```python
from build123d import *

# Parameters (mm, degrees)
F2_DEPTH = 12.7
F1_R     = 22.5055590266
F3_DEPTH = 7.62
F4_W     = 30.1420278847
F4_H     = 17.9640296847
F5_DEPTH = 2.54
F7_DEPTH = 1.27


with BuildPart() as f2:
    # F0 (on Front) → F2 (new body)
    with BuildSketch(Plane.XZ):
        Polygon((16.1803662777, 0), (37.0746999979, 0), (37.0746999979, 26.1179152876), (34.0169928968, 32.2333276272), (31.2140900642, 39.1131713986), (31.2140900642, 43.4449203312), (21.7861626297, 43.4449203312), (21.7861626297, 39.1131713986), (18.7284555286, 32.2333276272), (16.1803662777, 26.1179152876), align=None)
    extrude(amount=F2_DEPTH)


with BuildPart() as f3:
    # F1 (on Front) → F3 (new body)
    with BuildSketch(Plane.XZ):
        with Locations((78.2617554069, 32.2333276272)):
            Circle(F1_R)
    extrude(amount=F3_DEPTH)


with BuildPart() as f5:
    # F4 (on Top) → F5 (new body)
    with BuildSketch(Plane.XY):
        with Locations((-15.0710139424, 8.9820148423)):
            Rectangle(F4_W, F4_H)
    extrude(amount=F5_DEPTH)

    # F6 (on face) → F7 (join)
    with BuildSketch(Plane.XY.offset(2.54)):
        Polygon((-35.7478260994, 4.4591561891), (-30.1420278847, 2.4206847884), (0, 2.4206847884), (2.9831291176, 2.4206847884), (5.0216042437, 4.4591561891), (5.0216042437, 7.2620538995), (2.9831291176, 7.2620538995), (0, 7.2620538995), (-30.1420278847, 7.2620538995), (-32.6901189983, 7.2620538995), (-35.7478260994, 7.2620538995), align=None)
        Polygon((-30.1420278847, 11.8486145511), (0, 11.8486145511), (2.9831291176, 11.8486145511), (5.0216042437, 14.396703802), (0, 14.396703802), (-30.1420278847, 14.396703802), (-32.6901189983, 14.396703802), (-32.6901189983, 11.8486145511), align=None)
    extrude(amount=F7_DEPTH)


with BuildPart() as f12:
    # F11 (on Front) → F12 (revolve)
    with BuildSketch(Plane.XZ):
        with BuildLine():
            Line((0, -66.4687156677), (0, 55.9921823442))
            Line((0, 55.9921823442), (-22.0337584615, 55.9921823442))
            Line((-22.0337584615, 55.9921823442), (-35.9484543807, 45.556163555))
            ThreePointArc((-35.9484543807, 45.556163555), (-37.8180675739, 43.3159697459), (-38.4884551167, 40.476163003))
            Line((-38.4884551167, 40.476163003), (-38.4884551167, 26.2577953691))
            ThreePointArc((-38.4884551167, 26.2577953691), (-37.8180675121, 23.4179885028), (-35.9484541599, 21.1777946515))
            Line((-35.9484541599, 21.1777946515), (-32.1597233415, 18.3362476528))
            Line((-32.1597233415, 18.3362476528), (-37.2184558344, 11.5912683486))
            ThreePointArc((-37.2184558344, 11.5912683486), (-38.1625942485, 9.7893150524), (-38.4884551167, 7.7812693055))
            Line((-38.4884551167, 7.7812693055), (-38.4884551167, -21.9619643911))
            ThreePointArc((-38.4884551167, -21.9619643911), (-37.9697873011, -24.47554052), (-36.4985133985, -26.5784989984))
            Line((-36.4985133985, -26.5784989984), (-32.7925980091, -30.0785284489))
            Line((-32.7925980091, -30.0785284489), (-36.754989724, -34.2740041277))
            ThreePointArc((-36.754989724, -34.2740041277), (-38.0391963734, -36.2880546043), (-38.4884551167, -38.6340624095))
            Line((-38.4884551167, -38.6340624095), (-38.4884551167, -60.1187156677))
            ThreePointArc((-38.4884551167, -60.1187156677), (-36.6285831773, -64.6088437283), (-32.1384551167, -66.4687156677))
            Line((-32.1384551167, -66.4687156677), (0, -66.4687156677))
        make_face()
        with BuildLine():
            Line((0, 55.9921823442), (0, 67.4110209227))
            Line((0, 67.4110209227), (-20.4462584615, 67.4110209227))
            ThreePointArc((-20.4462584615, 67.4110209227), (-21.5687904766, 66.9460529378), (-22.0337584615, 65.8235209227))
            Line((-22.0337584615, 65.8235209227), (-22.0337584615, 55.9921823442))
            Line((-22.0337584615, 55.9921823442), (0, 55.9921823442))
        make_face()
    revolve(axis=Axis((0, 0, 0.4711526275), (0, 0, 1)))


solid = f12.part
```
Model file for the job. Use its own axes, mm. A direction names the side the tool comes from. Coordinates: 2 decimals unless noted, no trailing zeros. Write each loop counter-clockwise with the first axis right and the second up, starting at its lowest first coordinate (ties: lowest second). Pieces come first, ordered by that corner, then holes. Notation, with made-up numbers: (44.25, -14) - (89.25, -14) arc R20 cw to (89.25, -2) - close; hole circle Ø10 at (-21, 26). An arc over 180 degrees is marked (long way). One line per item, written item: value. Start each with the question number.
1. Mould opens along Z. For faces 4 (the flat face through (0, 0, 67.411)), 5 (the cylindrical face through (-36.7, -11.6, -7.3)), 6 (the conical face through (7.163, 32.255, -30.341)), 7 (the conical face through (-30.85, -9.715, 18.474)) say: released by +Z, released by -Z, zero draft, split by the parting line, or undercut.
2. Probe line 1 (Z direction, x = -21, y = -30.5); line 2 (Y direction, x = 11.5, z = -9.5); line 3 (Z direction, x = -20.5, y = 6.5). List the from-to ranges inside material, lowest first. Write a range as from..to.
3. Flat gauge pins, fed straight in: pin 1 (1.5 mm diameter, centred on x = 8.5, y = -26.5, fed in from +Z); pin 2 (6 mm diameter, centred on x = -17.5, y = -23.5, fed in from +Z); pin 3 (8 mm diameter, centred on x = 6, y = 28, fed in from +Z). Where does each tip first touch, or does it go through?
4. Slice it at C-C (z = -56.5). Write the cut outline in (x, y), plus the area to 3 significant figures.
5. Tool access for faces 1 (the flat face through (0, 0, -66.469)), 2 (the conical face through (4.3, -32.7, -29.9)), 3 (the cylindrical face through (-10.167, 19.548, 60.839)): list every direction of +Z, -Z, +X, -X, +Y, -Y with a clear straight run to the whole face (end or side of a thin tool).
Answers below:
1. face 4: released by +Z
1. face 5: zero draft
1. face 6: undercut
1. face 7: undercut
2. line 1: z = -64.17..-34.59, -26.01..11.84, 22.21..44.52
2. line 2: y = -36.73..36.73
2. line 3: z = -66.47..67.01
3. pin 1: stops at z = 52.21
3. pin 2: stops at z = 52.79
3. pin 3: stops at z = 54.04
4. outline: circle Ø76.98 at (0, 0)
4. area: 4,650 mm^2
5. face 1: -Z, +X, -X, +Y, -Y
5. face 2: none
5. face 3: +Z
